Check sheet for the modelled part. Datum: model origin and axes. Units: mm. A direction names the side the tool comes from. Round coordinates to 2 decimals unless told otherwise and drop trailing zeros. Loops run counter-clockwise (first coordinate to the right, second up) from the corner with the lowest first, then second, coordinate; pieces in that order, holes last. Notation, with made-up numbers: (-25.5, 55) - (9.5, 55) arc R5 ccw to (9.5, 62) - close; hole circle Ø6 at (-22, -37). An arc over 180 degrees is marked (long way). Return JSON: item names as keys, results as strings.
Autodesk Inventor part; units mm, degrees
ref_plane "YZ Plane" through (0, 0, 0) normal (1, 0, 0) x (0, 1, 0)
ref_plane "XZ Plane" through (0, 0, 0) normal (0, 1, 0) x (-1, 0, 0)
ref_plane "XY Plane" through (0, 0, 0) normal (0, 0, 1) x (1, 0, 0)
sketch "Sketch1" plane through (0, 0, 0) normal (0, 1, 0) x (-1, 0, 0)
  point P0 (0, 0)
sketch "Sketch2" plane through (0, 0, 0) normal (0, 1, 0) x (-1, 0, 0)
  line L0 (-19.9525, 52) -> (19.9525, 52)
  line L1 (19.9525, 52) -> (19.9525, -52)
  line L2 (19.9525, -52) -> (-19.9525, -52)
  line L3 (-19.9525, -52) -> (-19.9525, 52)
  line L4 (-19.9525, 52) -> (19.9525, -52) construction
  line L5 (19.9525, 52) -> (-19.9525, -52) construction
  circle A0 centre (13.4525, 45.5) radius 1.6
  circle A1 centre (-13.4525, 45.5) radius 1.6
  line L6 (0, 59.3125) -> (0, -64.5558)
  line L7 (36.5125, 0) -> (-39.6875, 0)
  circle A2 centre (13.4525, -45.5) radius 1.6
  circle A3 centre (-13.4525, -45.5) radius 1.6
  line L8 (0, -59.3125) -> (0, 64.5558)
  circle A4 centre (11, 8) radius 1.6
  circle A5 centre (-11, 8) radius 1.6
  circle A6 centre (-11, -32) radius 1.6
  circle A7 centre (11, -32) radius 1.6
  line L9 (-11, -8.25) -> (-20, -8.25)
  line L10 (-20, -20.75) -> (-11, -20.75)
  line L11 (-11, -20.75) -> (-11, -8.25)
  line L12 (-11, -8.25) -> (-20, -20.75) construction
  line L13 (-20, -8.25) -> (-11, -20.75) construction
  line L14 (-11, -8.25) -> (-19.9525, -8.25)
  line L15 (-19.9525, -8.25) -> (-19.9525, -20.75)
  line L16 (-19.9525, -20.75) -> (-11, -20.75)
  line L17 (-11, -20.75) -> (-11, -8.25)
  line L18 (11, -8.25) -> (20, -8.25)
  line L19 (20, -20.75) -> (11, -20.75)
  line L20 (11, -20.75) -> (11, -8.25)
  line L21 (11, -8.25) -> (20, -20.75) construction
  line L22 (20, -8.25) -> (11, -20.75) construction
  line L23 (11, -8.25) -> (19.9525, -8.25)
  line L24 (19.9525, -8.25) -> (19.9525, -20.75)
  line L25 (19.9525, -20.75) -> (11, -20.75)
  line L26 (11, -20.75) -> (11, -8.25)
  point P0 (0, 0)
  point P1 (-15.5, -14.5)
  point P2 (15.5, -14.5)
  point P3 (19.9525, -8.25)
  dimension "d0" = 104
  dimension "d1" = 39.905
  dimension "d2" = 3.2
  dimension "d3" = 3.2
  dimension "d5" = 6.5
  dimension "d7" = 6.5
  dimension "d11" = 3.2
  dimension "d12" = 3.2
  dimension "d13" = 11
  dimension "d14" = 11
  dimension "d15" = 8
  dimension "d16" = 8
  dimension "d17" = 3.2
  dimension "d18" = 3.2
  dimension "d19" = 40
  dimension "d20" = 40
  dimension "d21" = 11
  dimension "d22" = 11
  dimension "d23" = 12.5
  dimension "d24" = 9
  dimension "d25" = 8.25
  dimension "d26" = 11
  dimension "d27" = 6.5
  dimension "d28" = 6.5
extrude "Extrusion1" add sketch "Sketch2" along normal blind 3 contours L0 L6 L7 L3 | L0 L1 L7 L6 | L7 L6 L2 L3 L10 L11 L9 | L7 L1 L18 L20 L19 L2 L6
fillet "Fillet1" radius 4 4 edges at (19.9525, 1.5, 52) (-19.9525, 1.5, 52) (19.9525, 1.5, -52) (-19.9525, 1.5, -52)
sketch "Sketch3" plane through (0, 3, 0) normal (0, 1, 0) x (1, 0, 0)
  circle A0 centre (0, -0.0025) radius 10
  circle A1 centre (11, 32) radius 1.6
  circle A2 centre (-11, 32) radius 1.6
  circle A3 centre (-11, -8) radius 1.6
  circle A4 centre (11, -8) radius 1.6
  point P0 (0, 0)
  dimension "d35" = 13.6
  dimension "d36" = 13.6
properties part number "bottom"
Q1. Sectioned sample at A-A (z = 45.5). Enter the section's corners in (x, y).
Answer key:
{"outline": "(-19.95, 0) - (-15.05, 0) - (-15.05, 3) - (-19.95, 3) - close; (-11.85, 0) - (11.85, 0) - (11.85, 3) - (-11.85, 3) - close; (15.05, 0) - (19.95, 0) - (19.95, 3) - (15.05, 3) - close"}
Q2. Tool access check on faces 4 (the face through (15, 1, -8.25)), 5 (the face through (-9.4, 1.48, 7.93)), 6 (the face through (-15, 1, -8.25)). Record the directions out of +Z, -Z, +X, -X, +Y, -Y that give a thin tool (end or side, any length) a straight path to the whole face; none if there is none.
Answer key:
{"face 4": "+X, +Y, -Y", "face 5": "+Y, -Y", "face 6": "-X, +Y, -Y"}
Q3. Sectioned sample at B-B (y = 0.6). State how many separate pieces and enclosed holes the cut face has, plus the area to 3 significant figures.
Answer key:
{"separate pieces": "1", "enclosed holes": "8", "area": "3,850 mm²"}
Q4. Draft check along Z on faces 1 (the face through (0, 3, 1)), 2 (the face through (11, 1, -15)), 3 (the face through (18.81, 1.52, -50.8)). Enter one of: released by +Z, released by -Z, zero draft, split by the parting line, or undercut.
Answer key:
{"face 1": "zero draft", "face 2": "undercut", "face 3": "released by -Z"}
Q5. Sectioned sample at C-C (z = -17.5). Enter the section's corners in (x, y).
Answer key:
{"outline": "(-11, 0) - (11, 0) - (11, 3) - (-11, 3) - close"}
Q6. Depth check by flat-ended pin: P1, Ø5, axis at x = 13.45, z = 45.5, coming from the -Y side. Enter the tip coordinate at first touch or a pass-through.
Answer key:
{"P1": "stops at y = 0"}
Q7. Scan lines: probe 1 along Z at (x, y) = (12, 2.05); probe 2 along X at (y, z) = (0.45, 9); probe 3 along Z at (x, y) = (18, 2.05). Record each from-to range of solid material in increasing order. Write a range as [from, to].
Answer key:
{"probe 1": "z = [-52, -46.17], [-44.83, -33.25], [-30.75, -20.75], [-8.25, 6.75], [9.25, 44.83], [46.17, 52]", "probe 2": "x = [-19.95, -12.25], [-9.75, 9.75], [12.25, 19.95]", "probe 3": "z = [-51.44, -20.75], [-8.25, 51.44]"}
